Verification items for the finished model (mm, model axes). A direction names the side the tool comes from. Give positions to 0.01 mm unless a question says otherwise; leave off trailing zeros. Order: outer loops, then holes, each group sorted by start corner. A loop starts at its lowest first (then second) coordinate and runs counter-clockwise, first axis right, second up. Notation, with made-up numbers: (89, -10) - (107, -10) arc R35 ccw to (107, 28) - close; hole circle Ø9 at (-4, 32.25). An arc over 180 degrees is marked (long way). Answer as a JSON object with one key per item and string values.
```python
from build123d import *

# Parameters (mm, degrees)
F1_DEPTH = 40


with BuildPart() as f1:
    # F0 (on Top) → F1 (new body)
    with BuildSketch(Plane.XY):
        with BuildLine():
            ThreePointArc((-135, -87.75), (-131.485281, -96.235281), (-123, -99.75))
            Line((-123, -99.75), (123, -99.75))
            ThreePointArc((123, -99.75), (131.485281, -96.235281), (135, -87.75))
            Line((135, -87.75), (135, 81.331121))
            ThreePointArc((135, 81.331121), (132.403394, 88.429218), (125.839459, 92.17623))
            ThreePointArc((125.839459, 92.17623), (99.105981, 96.217898), (72.244569, 99.296609))
            ThreePointArc((72.244569, 99.296609), (67.790252, 98.888715), (63.794752, 96.877918))
            ThreePointArc((63.794752, 96.877918), (33.680622, 80.80401), (0, 75.25))
            ThreePointArc((0, 75.25), (-33.680622, 80.80401), (-63.794752, 96.877918))
            ThreePointArc((-63.794752, 96.877918), (-67.790252, 98.888715), (-72.244569, 99.296609))
            ThreePointArc((-72.244569, 99.296609), (-99.105981, 96.217898), (-125.839459, 92.17623))
            ThreePointArc((-125.839459, 92.17623), (-132.403394, 88.429218), (-135, 81.331121))
            Line((-135, 81.331121), (-135, -87.75))
        make_face()
    extrude(amount=F1_DEPTH)


solid = f1.part
```
(1) Material ranges on line 1 along Y through (x, z) = (35, 27); line 2 along Y through (x, z) = (19, 24); line 3 along X through (y, z) = (-90.5, 12.5), recorded low to high. Write a range as [from, to].
Computed values:
{"line 1": "y = [-99.75, 81.26]", "line 2": "y = [-99.75, 76.99]", "line 3": "x = [-134.68, 134.68]"}
(2) Gauge pin test, flat end, axial feed: pin 1 Ø5 at (x, z) = (20.5, 26) entering from +Y. Record the tip position at first contact, or that the pin passes through.
Computed values:
{"pin 1": "stops at y = 77.8"}
(3) Access from +Z, -Z, +X, -X, +Y, -Y to the whole of each face (thin tool, end or side, straight path). Record for faces 4 (the cylindrical face through (67.851, 98.906, 19.72)), 5 (the cylindrical face through (131.39, -96.33, 19.72)).
Computed values:
{"face 4": "+Z, -Z, +Y", "face 5": "+Z, -Z, +X, -Y"}
(4) Section check B-B (x = 32). Record the cut outline in (y, z), then the cut area to 3 significant figures.
Computed values:
{"outline": "(-99.75, 0) - (80.25, 0) - (80.25, 40) - (-99.75, 40) - close", "area": "7,200 mm²"}
(5) Section check A-A (z = 33). Record the cut outline in (x, y), then the cut area to 3 significant figures.
Computed values:
{"outline": "(-135, -87.75) arc R12 ccw to (-123, -99.75) - (123, -99.75) arc R12 ccw to (135, -87.75) - (135, 81.33) arc R11 ccw to (125.84, 92.18) arc R752.52 ccw to (72.24, 99.3) arc R12 ccw to (63.79, 96.88) arc R104.9 cw to (0, 75.25) arc R104.9 cw to (-63.79, 96.88) arc R12 ccw to (-72.24, 99.3) arc R752.52 ccw to (-125.84, 92.18) arc R11 ccw to (-135, 81.33) - close", "area": "51,000 mm²"}
(6) Section check C-C (x = -19). Record the cut outline in (y, z), then the cut area to 3 significant figures.
Computed values:
{"outline": "(-99.75, 0) - (76.99, 0) - (76.99, 40) - (-99.75, 40) - close", "area": "7,070 mm²"}
(7) Release check for a two-part mould opening along X. For faces 1 (the flat face through (135, -4, 20)), 2 (the cylindrical face through (-67.73, 98.87, 19.72)), 3 (the flat face through (-2, 1, 40)) record: pulls with the +X half, pulls with the -X half, needs draft (parallel to the pull), parting line crosses it, or undercut.
Computed values:
{"face 1": "pulls with the +X half", "face 2": "undercut", "face 3": "needs draft"}
